Geometry: see drawing. Coordinates: mm, zero at the bounding-box minimum. Give positions to 0.01 mm unless a question says otherwise; leave off trailing zeros. Write each loop counter-clockwise with the first axis right and the second up, starting at its lowest first coordinate (ties: lowest second). Pieces come first, ordered by that corner, then holes. Notation, with made-up numbers: M -9,4 L 13,4 A32 cw 13,33 Z; hole C -30.75,-28 d9. An arc over 180 degrees is marked long. Use a Markdown table: item, result. Add a question column.
1) Line query: line 1 (X direction, y = 3, z = 3); line 2 (Z direction, x = 3, y = 3.25); line 3 (Z direction, x = 7.25, y = 6.5). Output: solid intervals per line, ascending.
2) Pin query (flat end, axial travel): pin 1 (1.2 mm diameter, centred on x = 24, z = 16.5, fed in from +Y); pin 2 (1.2 mm diameter, centred on x = 24, z = 17, fed in from -Y). Return the tip coordinate at first contact, or that it passes through.
3) Section D-D on x = 16.5. Return the cut outline in (y, z).
4) Section C-C on y = 6. Return the cut outline in (x, z) (3 decimals).
5) Section B-B on z = 12.7. Return the cut outline in (x, y), then the cut area to 4 significant figures.
6) Section A-A on x = 3. Return the cut outline in (y, z).
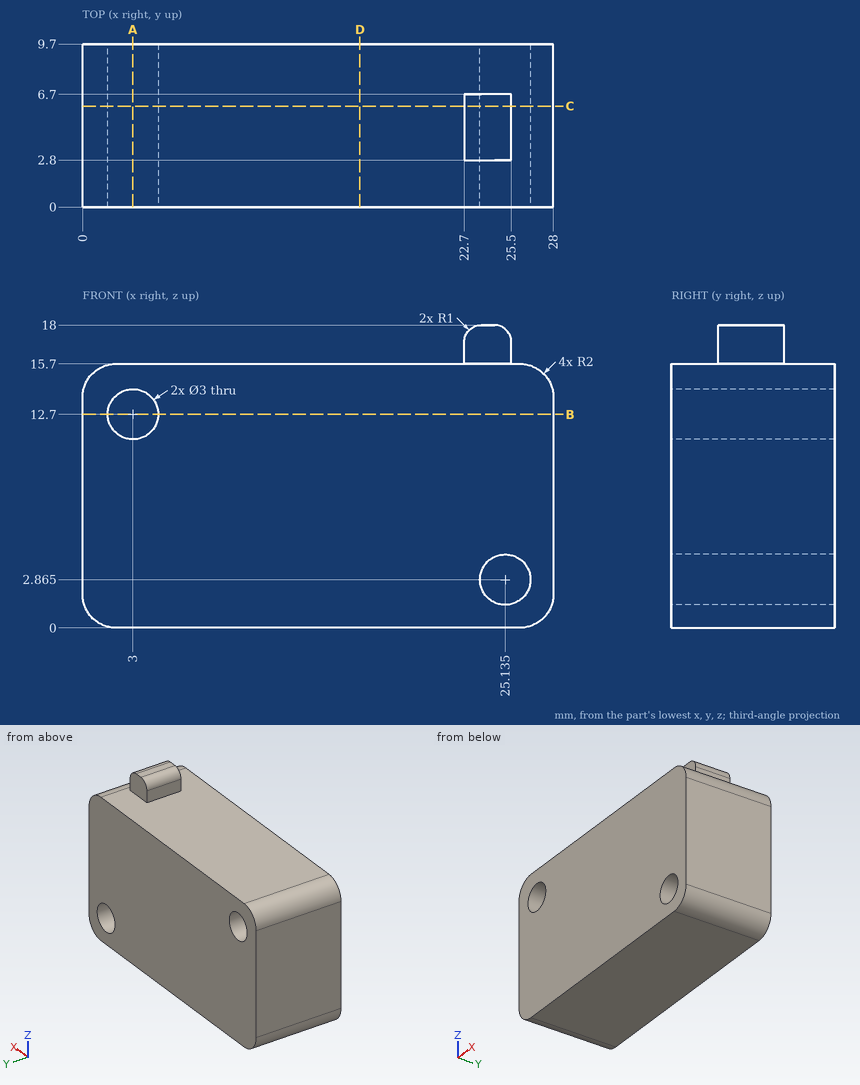
Found:
| question | item | result |
|---|---|---|
| 1 | line 1 | 0 to 23.64, 26.63 to 28 |
| 1 | line 2 | 0 to 11.2, 14.2 to 15.7 |
| 1 | line 3 | 0 to 15.7 |
| 2 | pin 1 | y = 6.7 |
| 2 | pin 2 | y = 2.8 |
| 3 | outline | M 0,0 L 9.7,0 L 9.7,15.7 L 0,15.7 Z |
| 4 | outline | M 0,2 A2 ccw 2,0 L 26,0 A2 ccw 28,2 L 28,13.7 A2 ccw 26,15.7 L 25.5,15.7 L 25.5,17 A1 ccw 24.5,18 L 23.7,18 A1 ccw 22.7,17 L 22.7,15.7 L 2,15.7 A2 ccw 0,13.7 Z; hole C 3,12.7 d3; hole C 25.135,2.865 d3 |
| 5 | outline | M 0,0 L 1.5,0 L 1.5,9.7 L 0,9.7 Z; M 4.5,0 L 28,0 L 28,9.7 L 4.5,9.7 Z |
| 5 | area | 242.5 mm² |
| 6 | outline | M 0,0 L 9.7,0 L 9.7,11.2 L 0,11.2 Z; M 0,14.2 L 9.7,14.2 L 9.7,15.7 L 0,15.7 Z |
